```python
from build123d import *

# Parameters (mm, degrees)
SKETCH1_R             = 90
BOSS_EXTRUDE1_DEPTH   = 13
SKETCH2_R             = 25
CUT_EXTRUDE1_DEPTH    = 128.941392833
SKETCH3_R             = 5.434212322
CUT_EXTRUDE2_DEPTH    = 11.967453
CIRPATTERN1_START     = 1.032546532
CIRPATTERN1_OUTLINE_R = 5.434212322
CIRPATTERN1_DEPTH     = 11.967453468


# Read off the part's stored shape, not the designer's step: CirPattern1
with BuildPart() as part:
    # Sketch1 → Boss-Extrude1 (new body)
    with BuildSketch(Plane(origin=(0, 0, 0), x_dir=(1, 0, 0), z_dir=(0, 1, 0))):
        with Locations(Location((0, 0, 0), (0, 0, 90))):
            Circle(SKETCH1_R)
    extrude(amount=BOSS_EXTRUDE1_DEPTH)

    # Sketch2 → Cut-Extrude1 (cut, through all)
    with BuildSketch(Plane(origin=(0, 0, 0), x_dir=(1, 0, 0), z_dir=(0, 1, 0))):
        with Locations(Location((0, 0, 0), (0, 0, 90))):
            Circle(SKETCH2_R)
    extrude(amount=CUT_EXTRUDE1_DEPTH, mode=Mode.SUBTRACT)

    # Sketch3 → Cut-Extrude2 (cut)
    with BuildSketch(Plane(origin=(0, 13, 0), x_dir=(1, 0, 0), z_dir=(0, 1, 0))):
        with Locations(Location((-33.896773813, 0, 0), (0, 0, 270))):
            Circle(SKETCH3_R)
    extrude(amount=-CUT_EXTRUDE2_DEPTH, mode=Mode.SUBTRACT)

    # CirPattern1 outline → CirPattern1 (cut)
    with BuildSketch(Plane(origin=(0, 0, 0), x_dir=(1, 0, 0), z_dir=(0, 1, 0)).offset(CIRPATTERN1_START)):
        with Locations((16.948386906, 29.355467228)):
            Circle(CIRPATTERN1_OUTLINE_R)
        with Locations((16.948386906, -29.355467228)):
            Circle(CIRPATTERN1_OUTLINE_R)
    extrude(amount=CIRPATTERN1_DEPTH, mode=Mode.SUBTRACT)


solid = part.part
```
Part model, mm, in its own coordinate system. A direction names the side the tool comes from. Round coordinates to 2 decimals unless told otherwise and drop trailing zeros. Loops run counter-clockwise (first coordinate to the right, second up) from the corner with the lowest first, then second, coordinate; pieces in that order, holes last.
1. Flat gauge pins, fed straight in: pin 1 (6.5 mm diameter, centred on x = -33.9, z = 0, fed in from +Y); pin 2 (8.5 mm diameter, centred on x = 19, z = 31, fed in from +Y); pin 3 (1 mm diameter, centred on y = 3, z = 5.5, fed in from +X); pin 4 (5 mm diameter, centred on x = 24.5, y = 10.5, fed in from +Z). Where does each tip first touch, or does it go through?
Solutions:
pin 1: stops at y = 1.03
pin 2: stops at y = 13
pin 3: stops at x = 89.86
pin 4: stops at z = 87.27
2. Slice it at B-B (z = 0). Give the cut face in (x, y).
Solutions:
outline: (-90, 0) - (-25, 0) - (-25, 13) - (-28.46, 13) - (-28.46, 1.03) - (-39.33, 1.03) - (-39.33, 13) - (-90, 13) - close; (25, 0) - (90, 0) - (90, 13) - (25, 13) - close
3. Slice it at C-C (y = 6.5). Give the cut face in (x, z).
Solutions:
outline: circle Ø180 at (0, 0); hole circle Ø10.87 at (-33.9, 0); hole circle Ø50 at (0, 0); hole circle Ø10.87 at (16.95, -29.36); hole circle Ø10.87 at (16.95, 29.36)
4. Slice it at A-A (x = 0). Give the cut face in (y, z), and give its area (3 significant figures).
Solutions:
outline: (0, -90) - (13, -90) - (13, -25) - (0, -25) - close; (0, 25) - (13, 25) - (13, 90) - (0, 90) - close
area: 1,690 mm2
5. Drill centre lines: line 1 along X through (y, z) = (4.5, 0); line 2 along Z through (x, y) = (13.5, 6); line 3 along Z through (x, y) = (2, 1). Where is each one in solid material? Low to high.
Solutions:
line 1: x = -90 to -39.33, -28.46 to -25, 25 to 90
line 2: z = -88.98 to -33.56, -25.16 to -21.04, 21.04 to 25.16, 33.56 to 88.98
line 3: z = -89.98 to -24.92, 24.92 to 89.98
6. 3-axis set-ups, long thin cutter, end or side, ignore diameter. For faces 4 (the face through (17, 1.033, 29)), 5 (the face through (-7.509, 6.409, -23.846)): which of +Z, -Z, +X, -X, +Y, -Y reach the whole face in a straight line?
Solutions:
face 4: +Y
face 5: +Y, -Y
7. Two-plate mould, pull along X, no slides. Class faces 1 (the face through (-34, 1.033, 0)), 2 (the face through (19, 0, -19)), 3 (the face through (34.471, 6.409, -83.137)): pulls with the +X half, pulls with the -X half, needs draft (parallel to the pull), parting line crosses it, or undercut.
Solutions:
face 1: undercut
face 2: needs draft
face 3: parting line crosses it
8. Slice it at D-D (x = 19.5). Give the cut face in (y, z).
Solutions:
outline: (0, -87.86) - (13, -87.86) - (13, -34.15) - (1.03, -34.15) - (1.03, -24.56) - (13, -24.56) - (13, -15.64) - (0, -15.64) - close; (0, 15.64) - (13, 15.64) - (13, 24.56) - (1.03, 24.56) - (1.03, 34.15) - (13, 34.15) - (13, 87.86) - (0, 87.86) - close
